Autodesk Inventor part; units mm, degrees
ref_plane "YZ Plane" through (0, 0, 0) normal (1, 0, 0) x (0, 1, 0)
ref_plane "XZ Plane" through (0, 0, 0) normal (0, 1, 0) x (-1, 0, 0)
ref_plane "XY Plane" through (0, 0, 0) normal (0, 0, 1) x (1, 0, 0)
sketch "Sketch1" plane through (0, 0, 0) normal (0, 0, 1) x (1, 0, 0)
  circle A0 centre (0, 0) radius 41.148
  dimension "d0" = 82.296
extrude "Extrusion1" add sketch "Sketch1" against normal blind 68.072
sketch "Sketch2" plane through (0, 0, 0) normal (0, 0, 1) x (1, 0, 0)
  circle A0 centre (0, 0) radius 9.525
  dimension "d3" = 19.05
extrude "Extrusion2" cut sketch "Sketch2" against normal blind 68.072
sketch "Sketch3" plane through (0, 0, -68.072) normal (0, 0, -1) x (-1, 0, 0)
  circle A0 centre (0, 0) radius 21.844
  dimension "d6" = 43.688
extrude "Extrusion3" cut sketch "Sketch3" against normal blind 23.622
sketch "Sketch4" plane through (0, 0, 0) normal (0, 0, 1) x (1, 0, 0)
  circle A0 centre (0, 0) radius 9.525
extrude "Extrusion4" add sketch "Sketch4" against normal blind 6.35
loft "Loft1" cut section 1 edges at (-9.525, 0, -6.35) section 2 edges at (21.844, 0, -44.45)
sketch "Sketch5" plane through (0, 0, 0) normal (0, 0, 1) x (1, 0, 0)
  point P0 (0, 0)
hole "Hole1" at (0, 0, 0) direction (0, 0, -1) diameter 19.05 depth 50.419 tip angle 118
sketch "Sketch6" plane through (0, 0, 0) normal (0, 0, 1) x (1, 0, 0)
  circle A0 centre (0, 0) radius 41.148
  circle A1 centre (0, 0) radius 31.75
  dimension "d22" = 63.5
sketch "Sketch7" plane through (0, 0, -68.072) normal (0, 0, -1) x (-1, 0, 0)
  circle A0 centre (0, 0) radius 41.148
  circle A1 centre (0, 0) radius 9.525
  circle A2 centre (0, 0) radius 28.575
  dimension "d23" = 57.15
extrude "Extrusion5" cut sketch "Sketch7" against normal blind 23.622 contours A0
extrude "Extrusion6" cut sketch "Sketch6" against normal blind 38.1
sketch "Sketch8" plane through (0, 0, 0) normal (0, 0, 1) x (1, 0, 0)
  circle A0 centre (0, 0) radius 31.75
  circle A1 centre (0, 0) radius 41.148
extrude "Extrusion7" add sketch "Sketch8" against normal blind 6.35
sketch "Sketch9" plane through (0, 0, 0) normal (0, 0, 1) x (1, 0, 0)
  circle A0 centre (0, 36.449) radius 2.3812
  circle A1 centre (31.5658, 18.2245) radius 2.3812
  circle A2 centre (31.5658, -18.2245) radius 2.3812
  circle A3 centre (0, -36.449) radius 2.3812
  circle A4 centre (-31.5658, -18.2245) radius 2.3812
  circle A5 centre (-31.5658, 18.2245) radius 2.3812
  point P0 (0, 0)
  dimension "d30" = 4.7625
  dimension "d33" = 360
extrude "Extrusion8" cut sketch "Sketch9" against normal blind 127
properties part number "PreCombChamber4_4"
Model file for the job. Use its own axes, mm. A direction names the side the tool comes from. Coordinates: 2 decimals unless noted, no trailing zeros. Write each loop counter-clockwise with the first axis right and the second up, starting at its lowest first coordinate (ties: lowest second). Pieces come first, ordered by that corner, then holes. Notation, with made-up numbers: (16.25, 15.5) - (45.25, 15.5) arc R19 ccw to (45.25, 22.5) - close; hole circle Ø3 at (-9, 40.5). An arc over 180 degrees is marked (long way). One line per question, with ' | ' between items. Start each with the question number.
Q1. Drill centre lines: line 1 (Z direction, x = 19, y = 27); line 2 (Y direction, x = -31, z = -5); line 3 (Y direction, x = -6, z = -30). Where is each one in solid material? Low to high. Write a range as [from, to].
Q2. Cut at C-C, the plane x = 0. Give the number of separate pieces and of enclosed holes in the cut face, then the cut area to 3 significant figures.
Q3. Cut at D-D, the plane z = -15.5. List the corners of the cut face in (x, y).
Q4. Cut at B-B, the plane y = 26. List the corners of the cut face in (x, z).
Q5. Cut at A-A, the plane z = -60.5. List the corners of the cut face in (x, y) (3 decimals), then the cut area to 3 significant figures.
Q6. Pull direction X, two halves, no side cores. Call faces 4 (the face through (5.796, 7.559, -3.219)), 5 (the face through (-9, 31, -38.1)), 6 (the face through (-29.366, 17.312, -3.131)), 7 (the face through (-6.883, -30.995, -22.003)): pulls with the +X half, pulls with the -X half, needs draft (parallel to the pull), parting line crosses it, or undercut.
Q7. 3-axis set-ups, long thin cutter, end or side, ignore diameter. For faces 1 (the face through (-9, 31, -6.35)), 2 (the face through (-9, 28, -44.45)), 3 (the face through (-29.295, -17.509, -41.231)): which of +Z, -Z, +X, -X, +Y, -Y reach the whole face in a straight line?
Q8. Pin check, flat tips, straight feed: pin 1 (12 mm diameter, centred on y = -2, z = -12.5, fed in from -X); pin 2 (5 mm diameter, centred on y = 22.5, z = -20.5, fed in from -X); pin 3 (4 mm diameter, centred on x = -1.5, z = -37.5, fed in from +Y). Stop position of each tip, or through.
Answer below:
1) line 1: [-44.45, -38.1], [-6.35, 0] | line 2: [-27.06, -20.54], [-15.91, 15.91], [20.54, 27.06] | line 3: [-31.18, -16.09], [16.09, 31.18]
2) separate pieces: 6 | enclosed holes: 0 | area: 1,940 mm^2
3) outline: circle Ø63.5 at (0, 0); hole circle Ø24.97 at (0, 0)
4) outline: (-31.89, -44.45) - (-11.85, -44.45) - (-11.85, -68.07) - (11.85, -68.07) - (11.85, -44.45) - (31.89, -44.45) - (31.89, -38.1) - (18.22, -38.1) - (18.22, -6.35) - (31.89, -6.35) - (31.89, 0) - (-31.89, 0) - (-31.89, -6.35) - (-18.22, -6.35) - (-18.22, -38.1) - (-31.89, -38.1) - close
5) outline: circle Ø57.15 at (0, 0); hole circle Ø43.688 at (0, 0) | area: 1,070 mm^2
6) face 4: undercut | face 5: needs draft | face 6: undercut | face 7: parting line crosses it
7) face 1: none | face 2: -Z | face 3: +Z, -Z
8) pin 1: x = -31.75 | pin 2: x = -24.66 | pin 3: y = 41.15
